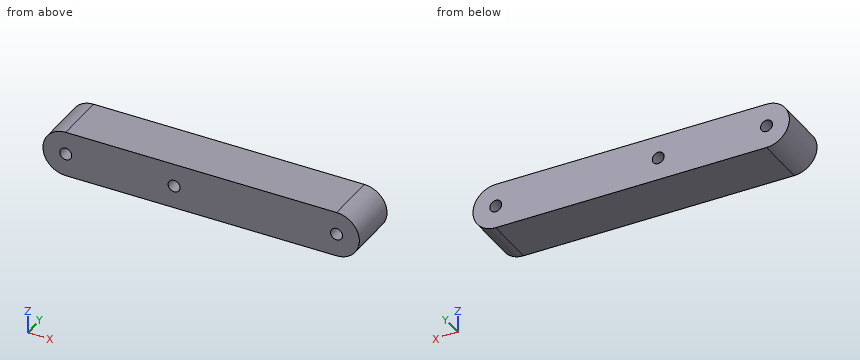
```python
from build123d import *

# Parameters (mm, degrees)
EXTRUDE_1_DEPTH     = 9
SKETCH_3_R          = 1.05
CUT_EXTRUDE_1_DEPTH = 9


with BuildPart() as part:
    # 草图2 → 凸台-拉伸1 (new body)
    with BuildSketch(Plane(origin=(0, 0, 0), x_dir=(1, 0, 0), z_dir=(0, 1, 0))):
        with BuildLine():
            Line((0, 0), (47.5, 0))
            ThreePointArc((47.5, 0), (51.5, -4), (47.5, -8))
            Line((47.5, -8), (0, -8))
            ThreePointArc((0, -8), (-4, -4), (0, 0))
        make_face()
    extrude(amount=EXTRUDE_1_DEPTH)

    # 草图3 → 切除-拉伸1 (cut)
    with BuildSketch(Plane.XZ):
        with Locations((0, 4)):
            Circle(SKETCH_3_R)
        with Locations((19, 4)):
            Circle(SKETCH_3_R)
        with Locations((47.5, 4)):
            Circle(SKETCH_3_R)
    extrude(amount=-CUT_EXTRUDE_1_DEPTH, mode=Mode.SUBTRACT)


solid = part.part
```
Could you check a few things on this model? Use its own coordinates, in mm. Round coordinates to 2 decimals unless told otherwise and drop trailing zeros. Loops run counter-clockwise (first coordinate to the right, second up) from the corner with the lowest first, then second, coordinate; pieces in that order, holes last.
Q1. Please list where these lines run through material, in increasing order: L1, parallel to Z at x = 47.5, y = 3.25; L2, parallel to X at y = 3.25, z = 3.25; L3, parallel to X at y = 2.75, z = 3.5.
Q2. I want a section at A-A (x = 19). Write out the boundary of the cut face in (y, z).
Q3. For P1, Ø3.5, axis at x = 47.5, z = 4, coming from the -Y side, with a flat end and sliding along its axis, tell me the tip position at first contact or that it passes through.
Q4. I want a section at B-B (z = 4). Write out the boundary of the cut face in (x, y).
Q5. I want a section at C-C (y = 7.75). Write out the boundary of the cut face in (x, z).
Q6. I want a section at D-D (z = 6). Write out the boundary of the cut face in (x, y), and give its area (3 significant figures).
Answer below:
1. L1: z = 0 to 2.95, 5.05 to 8
1. L2: x = -3.93 to -0.73, 0.73 to 18.27, 19.73 to 46.77, 48.23 to 51.43
1. L3: x = -3.97 to -0.92, 0.92 to 18.08, 19.92 to 46.58, 48.42 to 51.47
2. outline: (0, 0) - (9, 0) - (9, 2.95) - (0, 2.95) - close; (0, 5.05) - (9, 5.05) - (9, 8) - (0, 8) - close
3. P1: stops at y = 0
4. outline: (-4, 0) - (-1.05, 0) - (-1.05, 9) - (-4, 9) - close; (1.05, 0) - (17.95, 0) - (17.95, 9) - (1.05, 9) - close; (20.05, 0) - (46.45, 0) - (46.45, 9) - (20.05, 9) - close; (48.55, 0) - (51.5, 0) - (51.5, 9) - (48.55, 9) - close
5. outline: (0, 0) - (47.5, 0) arc R4 ccw to (47.5, 8) - (0, 8) arc R4 ccw to start; hole circle Ø2.1 at (0, 4); hole circle Ø2.1 at (19, 4); hole circle Ø2.1 at (47.5, 4)
6. outline: (-3.46, 0) - (50.96, 0) - (50.96, 9) - (-3.46, 9) - close
6. area: 490 mm2
